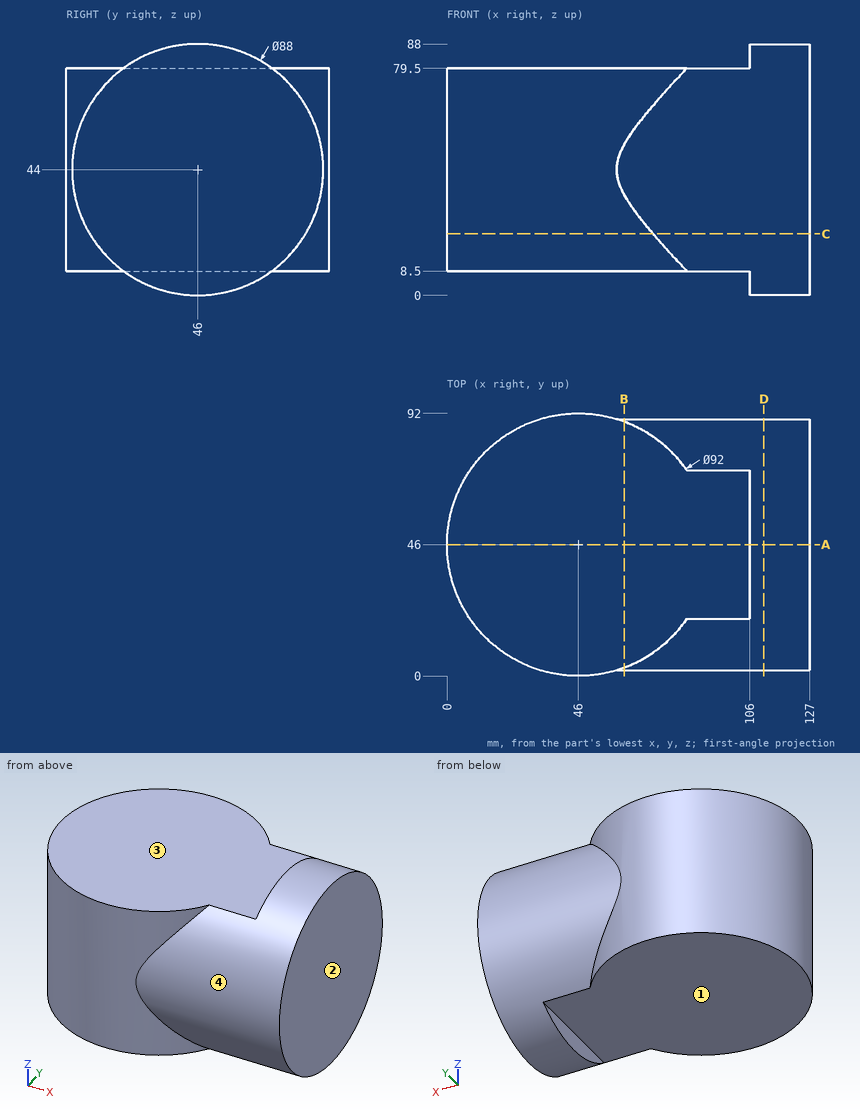
Can you work these out from the drawing? Everything is in mm from the part's minimum corner. A direction names the side the tool comes from. Give positions to 0.01 mm unless a question says otherwise; leave off trailing zeros. Loops run counter-clockwise (first coordinate to the right, second up) from the corner with the lowest first, then second, coordinate; pieces in that order, holes last. Notation, with made-up numbers: M 54,67 L 104,67 A5 ccw 104,75 Z; hole C -38,45 d9. An arc over 180 degrees is marked long. Use CSV: the item, a comma, the result in double quotes. Start each with the question number.
1. On a 3-axis mill with a long thin cutter (end or side, diameter ignored), from which of +Z, -Z, +X, -X, +Y, -Y can I reach the whole of each face in a straight line? I mean the marked faces 1, 2, 3 and 4. Say none if no direction works.
2. If I drill on L1, parallel to Z at x = 46.5, y = 21.5; L2, parallel to X at y = 58, z = 80; L3, parallel to Y at x = 12.5, z = 34, over which ranges is the centre line in solid material (lowest first)?
3. Imagine slicing it at C-C, the plane z = 21.5. Write out the boundary of the cut face in (x, y), plus the area to 3 significant figures.
4. Imagine slicing it at B-B, the plane x = 62. Write out the boundary of the cut face in (y, z).
5. Imagine slicing it at D-D, the plane x = 111. Write out the boundary of the cut face in (y, z).
6. Imagine slicing it at A-A, the plane y = 46. Write out the boundary of the cut face in (x, z), plus the area to 3 significant figures.
7. For P1, Ø6, axis at x = 48, y = 31, coming from the +Z side; P2, Ø12, axis at x = 77.5, z = 47, coming from the +Y side; P3, Ø7, axis at y = 46, z = 85, coming from the -X side, each with a flat end and sliding along its axis, tell me the tip position at first contact or that it passes through.
Response values:
1,face 1,"-Z, -X, +Y, -Y"
1,face 2,"+Z, -Z, +X, +Y, -Y"
1,face 3,"+Z, -X, +Y, -Y"
1,face 4,"+X"
2,L1,"8.5 to 79.5"
2,L2,"106 to 127"
2,L3,"14.48 to 77.52"
3,outline,"M 72.2,8.19 L 127,8.19 L 127,83.81 L 72.2,83.81 A46 ccw long Z"
3,area,"9,740 mm^2"
4,outline,"M 2.87,8.5 L 89.13,8.5 L 89.13,35.28 A44 ccw 89.13,52.72 L 89.13,79.5 L 2.87,79.5 L 2.87,52.72 A44 ccw 2.87,35.28 Z"
5,outline,"C 46,44 d88"
6,outline,"M 0,8.5 L 106,8.5 L 106,0 L 127,0 L 127,88 L 106,88 L 106,79.5 L 0,79.5 Z"
6,area,"9,370 mm^2"
7,P1,"z = 79.5"
7,P2,"y = 90"
7,P3,"x = 106"
